Autodesk Inventor part; units mm, degrees
ref_plane "YZ Plane" through (0, 0, 0) normal (1, 0, 0) x (0, 1, 0)
ref_plane "XZ Plane" through (0, 0, 0) normal (0, 1, 0) x (-1, 0, 0)
ref_plane "XY Plane" through (0, 0, 0) normal (0, 0, 1) x (1, 0, 0)
sketch "Sketch1" plane through (0, 0, 0) normal (0, 0, 1) x (1, 0, 0)
  line L0 (49.2125, 0) -> (54.6328, 0)
  line L1 (357.1875, 0) -> (350.9902, 0)
  arc A0 (0, 49.2125) -> (65.0875, 2.6308) centre (49.2125, 49.2125) ccw
  arc A1 (345.2239, 1.4763) -> (406.4, 49.2125) centre (357.1875, 49.2125) ccw
  arc A2 (203.2, 19.05) -> (54.6328, 0) centre (202.8115, -566.7686) ccw
  arc A3 (350.9902, 0) -> (345.2239, 1.4763) centre (202.8115, -566.7686) ccw
  arc A4 (65.0875, 2.6308) -> (54.6328, 0) centre (202.8115, -566.7686) ccw
  arc A5 (350.9902, 0) -> (203.2, 19.05) centre (202.8115, -566.7686) ccw
  line L2 (0, 49.2125) -> (0, 228.6)
  line L3 (406.4, 228.6) -> (406.4, 49.2125)
  line L4 (0, 228.6) -> (406.4, 228.6)
  point P0 (0, 0)
  point P1 (57.0671, 0.6309)
extrude "Extrusion1" add sketch "Sketch1" along normal blind 5.5563 contours A0 L2 L4 L3 A1 A5 A2
sketch "Sketch2" plane through (0, 0, 5.5563) normal (0, 0, 1) x (1, 0, 0)
  arc A0 (0, 49.2125) -> (57.0671, 0.6309) centre (49.2125, 49.2125) ccw
  arc A1 (345.2239, 1.4763) -> (406.4, 49.2125) centre (357.1875, 49.2125) ccw
  line L0 (361.7622, 0.2131) -> (361.7412, 44.6631)
  line L1 (361.7412, 44.6631) -> (406.1912, 44.6631)
  line L2 (0.2109, 44.6609) -> (44.6609, 44.6609)
  line L3 (44.6609, 44.6609) -> (44.6609, 0.2109)
  line L4 (365.2681, 38.3131) -> (368.9342, 44.6631)
  line L5 (365.2681, 51.0131) -> (368.9342, 44.6631)
  line L6 (357.9357, 51.0131) -> (365.2681, 51.0131)
  line L7 (357.9357, 38.3131) -> (365.2681, 38.3131)
  line L8 (357.9357, 51.0131) -> (354.2695, 44.6631)
  line L9 (354.2695, 44.6631) -> (357.9357, 38.3131)
  line L10 (48.1878, 38.3109) -> (51.854, 44.6609)
  line L11 (48.1878, 51.0109) -> (51.854, 44.6609)
  line L12 (40.8554, 51.0109) -> (48.1878, 51.0109)
  line L13 (40.8554, 38.3109) -> (48.1878, 38.3109)
  line L14 (40.8554, 51.0109) -> (37.1893, 44.6609)
  line L15 (37.1893, 44.6609) -> (40.8554, 38.3109)
  circle A2 centre (361.7412, 44.6631) radius 2.9337
  circle A3 centre (44.6609, 44.6609) radius 2.9337
  point P0 (0, 0)
  dimension "d97" = 44.45
  dimension "d99" = 44.45
  dimension "d100" = 44.45
  dimension "d101" = 44.45
  dimension "d102" = 12.7
  dimension "d103" = 12.7
  dimension "d104" = 12.7
  dimension "d105" = 7.3323
  dimension "d106" = 7.3323
  dimension "d107" = 7.3323
  dimension "d108" = 7.3323
  dimension "d109" = 7.3323
  dimension "d110" = 7.3323
  dimension "d111" = 12.7
  dimension "d112" = 12.7
  dimension "d113" = 12.7
  dimension "d114" = 7.3323
  dimension "d115" = 7.3323
  dimension "d116" = 7.3323
  dimension "d117" = 7.3323
  dimension "d118" = 7.3323
  dimension "d119" = 7.3323
  dimension "d145" = 5.8674
  dimension "d156" = 5.8674
extrude "Extrusion2" cut sketch "Sketch2" against normal through all contours A3 L3 L2 | L2 L3 A3 | A2 L1 L0 | L0 L1 A2
sketch "Sketch5" plane through (-0.198, 12.7962, 5.5563) normal (0, 0, 1) x (1, 0, 0)
  circle A0 centre (31.948, 184.0538) radius 2.9337
  circle A1 centre (374.848, 184.0538) radius 2.9337
  line L0 (31.948, 184.0538) -> (203.398, 184.0538)
  circle A2 centre (203.398, 184.0538) radius 2.9337
  point P0 (0.198, 215.8038)
  dimension "d141" = 5.8674
  dimension "d140" = 5.8674
  dimension "d139" = 171.45
  dimension "d138" = 5.8674
extrude "Extrusion6" cut sketch "Sketch5" against normal up to surface (5.5563 mm away)
sketch "Sketch6" plane through (0, 0, 5.5563) normal (0, 0, 1) x (1, 0, 0)
  ellipse E0 centre (293.3334, 94.2801) end of major axis (293.3295, 96.2801) minor radius 2
  ellipse E1 centre (293.3643, 62.2802) end of major axis (293.3569, 64.2802) minor radius 2
  circle A0 centre (361.7412, 44.6631) radius 2.9337
  line L0 (361.7412, 44.6631) -> (293.3643, 44.6631)
  line L1 (293.3643, 44.6631) -> (293.3643, 62.2802)
  ellipse E2 centre (113.007, 94.278) end of major axis (113.0032, 96.278) minor radius 2
  ellipse E3 centre (113.0379, 62.2781) end of major axis (113.0305, 64.2781) minor radius 2
  line L2 (113.0379, 44.6609) -> (113.0379, 62.2781)
  circle A1 centre (293.3643, 78.2802) radius 4.699
  circle A2 centre (113.0379, 78.278) radius 4.699
  circle A3 centre (44.6609, 44.6609) radius 2.9337
  line L3 (44.6609, 44.6609) -> (113.0379, 44.6609)
  point P0 (0, 0)
  dimension "d147" = 17.6171
  dimension "d148" = 68.3769
  dimension "d150" = 17.6171
  dimension "d152" = 9.398
  dimension "d153" = 9.398
  dimension "d157" = 68.3769
extrude "Extrusion7" cut sketch "Sketch6" against normal through all contours A1 | A2
properties part number "FTC Outside Panels" material "Wood (Oak)"
CAD build for the part. Positions are in the model's coordinates, mm. A direction names the side the tool comes from. Give positions to 0.01 mm unless a question says otherwise; leave off trailing zeros. Order: outer loops, then holes, each group sorted by start corner. A loop starts at its lowest first (then second) coordinate and runs counter-clockwise, first axis right, second up.
(1) Mould opens along Y. For faces 1 (the cylindrical face through (17.768, 11.356, 2.739)), 2 (the cylindrical face through (117.52, 79.69, 2.82)), 3 (the cylindrical face through (297.705, 76.48, 2.817)), 4 (the flat face through (200, 116, 0)) say: released by +Y, released by -Y, zero draft, split by the parting line, or undercut.
(2) Drill centre lines: L1, parallel to Y at x = 199.5, z = 2; L2, parallel to Y at x = 43, z = 1.45; L3, parallel to X at y = 76.5, z = 3.25. Where is each one in solid material? Low to high.
(3) Tool access for faces 5 (the flat face through (200, 116, 5.556)), 6 (the cylindrical face through (128.53, 14.32, 2.74)): list every direction of +Z, -Z, +X, -X, +Y, -Y with a clear straight run to the whole face (end or side of a thin tool).
(4) Saw through at B-B, the plane y = 29. Give the cut face in (x, z).
(5) Saw through at C-C, the plane x = 259.5. Give the cut face in (y, z), then the cut area to 3 significant figures.
(6) Saw through at A-A, the plane z = 3. State how many separate pieces and enclosed holes the cut face has, then the cut area to 3 significant figures.
(7) Flat gauge pins, fed straight in: pin 1 (1.5 mm diameter, centred on x = 178, z = 4.5, fed in from -Y); pin 2 (4.5 mm diameter, centred on x = 374.65, y = 196.85, fed in from -Z). Where does each tip first touch, or does it go through?
Results found:
1. face 1: released by -Y
1. face 2: undercut
1. face 3: undercut
1. face 4: zero draft
2. L1: y = 19.04 to 228.6
2. L2: y = 0.39 to 42.24, 47.08 to 228.6
2. L3: x = 0 to 108.69, 117.39 to 289.02, 297.71 to 406.4
3. face 5: +Z, +X, -X, +Y, -Y
3. face 6: +Z, -Z, -Y
4. outline: (4.34, 0) - (402.06, 0) - (402.06, 5.56) - (4.34, 5.56) - close
5. outline: (16.3, 0) - (228.6, 0) - (228.6, 5.56) - (16.3, 5.56) - close
5. area: 1,180 mm2
6. separate pieces: 1
6. enclosed holes: 7
6. area: 87,800 mm2
7. pin 1: stops at y = 18.49
7. pin 2: passes through
